Input: part model. Units: mm. Frame: model coordinates. A direction names the side the tool comes from. Coordinates: 2 decimals unless noted, no trailing zeros. Order: outer loops, then holes, each group sorted by start corner. A loop starts at its lowest first (then second) coordinate and runs counter-clockwise, first axis right, second up. Notation, with made-up numbers: (44, 60) -> (74, 60) arc R22 ccw to (74, 77) -> close; hole circle Ø11 at (35.5, 25.25). An arc over 180 degrees is marked (long way). Write each question's results on one line, items separated by ' | '.
```python
from build123d import *

# Parameters (mm, degrees)
F0_W     = 7.9375
F0_H     = 34.493074
F0_R     = 1.7272
F1_DEPTH = 25.4
F2_R     = 1.35255
F3_DEPTH = 4.7625
F4_R     = 1.35255
F5_DEPTH = 4.7625


with BuildPart() as f1:
    # F0 (on Top) → F1 (new body)
    with BuildSketch(Plane.XY):
        Rectangle(F0_W, F0_H)
        Circle(F0_R, mode=Mode.SUBTRACT)
    extrude(amount=F1_DEPTH)

    # F2 (on face) → F3 (cut)
    with BuildSketch(Plane(origin=(0, 17.246537, 0), x_dir=(-1, 0, 0), z_dir=(0, 1, 0))):
        with Locations((0, 3.96875)):
            Circle(F2_R)
        with Locations((0, 21.43125)):
            Circle(F2_R)
    extrude(amount=-F3_DEPTH, mode=Mode.SUBTRACT)

    # F4 (on face) → F5 (cut)
    with BuildSketch(Plane.XZ.offset(17.246537)):
        with Locations((0, 21.43125)):
            Circle(F4_R)
        with Locations((0, 3.96875)):
            Circle(F4_R)
    extrude(amount=-F5_DEPTH, mode=Mode.SUBTRACT)


solid = f1.part
```
(1) Cut plane B-B, the plane y = 0. Return loops of the section in (x, z), plus the area to 3 significant figures.
Return value:
outline: (-3.97, 0) -> (-1.73, 0) -> (-1.73, 25.4) -> (-3.97, 25.4) -> close; (1.73, 0) -> (3.97, 0) -> (3.97, 25.4) -> (1.73, 25.4) -> close | area: 114 mm2
(2) Cut plane A-A, the plane x = 0. Return loops of the section in (y, z).
Return value:
outline: (-17.25, 0) -> (-1.73, 0) -> (-1.73, 25.4) -> (-17.25, 25.4) -> (-17.25, 22.78) -> (-12.48, 22.78) -> (-12.48, 20.08) -> (-17.25, 20.08) -> (-17.25, 5.32) -> (-12.48, 5.32) -> (-12.48, 2.62) -> (-17.25, 2.62) -> close; (1.73, 0) -> (17.25, 0) -> (17.25, 2.62) -> (12.48, 2.62) -> (12.48, 5.32) -> (17.25, 5.32) -> (17.25, 20.08) -> (12.48, 20.08) -> (12.48, 22.78) -> (17.25, 22.78) -> (17.25, 25.4) -> (1.73, 25.4) -> close
(3) Reachability of faces 4 (the face through (0, -12.484, 21)), 5 (the face through (-2, 0, 0)), 6 (the face through (-0.62, 14.9, 20.23)) from +Z, -Z, +X, -X, +Y, -Y: full face, straight path, thin tool, end or side. Return the list, or none.
Return value:
face 4: -Y | face 5: -Z, +X, -X, +Y, -Y | face 6: +Y
(4) Mould query, pull axis Y, two halves, no side actions, for faces 1 (the face through (0, 17.247, 13)), 2 (the face through (0, -17.247, 13)), 3 (the face through (-0.225, 1.713, 12.522)). Classes: +Y half, -Y half, draft (parallel to the pull), parting line (faces both ways), or undercut.
Return value:
face 1: +Y half | face 2: -Y half | face 3: undercut
(5) Cut plane D-D, the plane z = 3. Return loops of the section in (x, y).
Return value:
outline: (-3.97, -17.25) -> (-0.94, -17.25) -> (-0.94, -12.48) -> (0.94, -12.48) -> (0.94, -17.25) -> (3.97, -17.25) -> (3.97, 17.25) -> (0.94, 17.25) -> (0.94, 12.48) -> (-0.94, 12.48) -> (-0.94, 17.25) -> (-3.97, 17.25) -> close; hole circle Ø3.45 at (0, 0)
(6) Cut plane C-C, the plane z = 20.5. Return loops of the section in (x, y).
Return value:
outline: (-3.97, -17.25) -> (-0.98, -17.25) -> (-0.98, -12.48) -> (0.98, -12.48) -> (0.98, -17.25) -> (3.97, -17.25) -> (3.97, 17.25) -> (0.98, 17.25) -> (0.98, 12.48) -> (-0.98, 12.48) -> (-0.98, 17.25) -> (-3.97, 17.25) -> close; hole circle Ø3.45 at (0, 0)
(7) Line query: line 1 along Z through (x, y) = (0, 15.95); line 2 along Z through (x, y) = (-0.5, -13.5); line 3 along Y through (x, z) = (0, 23.75). Output: solid intervals per line, ascending. Write a range as from..to.
Return value:
line 1: 0..2.62, 5.32..20.08, 22.78..25.4 | line 2: 0..2.71, 5.23..20.17, 22.69..25.4 | line 3: -17.25..-1.73, 1.73..17.25
(8) Pin query (flat end, axial travel): P1, Ø2, axis at x = 0, z = 21.43, coming from the +Y side; P2, Ø0.8, axis at x = -0.5, z = 4.5, coming from the -Y side. Return the tip coordinate at first contact, or that it passes through.
Return value:
P1: y = 12.48 | P2: y = -12.48
